Build history of the part. All positions in model axes, mm. Face numbers are marked on the shaded views. A direction names the side the tool comes from. Round coordinates to 2 decimals unless told otherwise and drop trailing zeros. Loops run counter-clockwise (first coordinate to the right, second up) from the corner with the lowest first, then second, coordinate; pieces in that order, holes last.
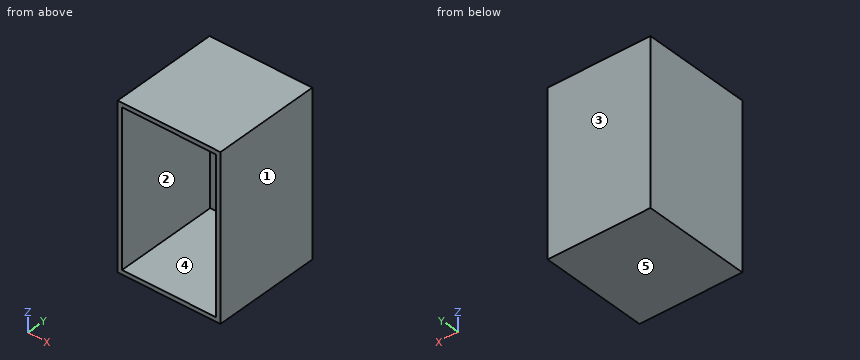
from build123d import *

# Parameters (mm, degrees)
F0_W     = 81.1607763171
F0_H     = 89.4276052713
F1_DEPTH = 381
F2_DEPTH = 482.6
F3_DEPTH = 279.4
F4_T     = -15.24


with BuildPart() as f1:
    # F0 (on Front) → F1 (new body)
    with BuildSketch(Plane.XZ):
        Rectangle(F0_W, F0_H)
    extrude(amount=F1_DEPTH)

    # F2 (add): a face of the model
    f2_faces = [f1.faces().sort_by_distance(p)[0] for p in [
        (0, -190.5, 44.7138026357),
    ]]
    extrude(f2_faces, amount=F2_DEPTH)

    # F3 (add): a face of the model
    f3_faces = [f1.faces().sort_by_distance(p)[0] for p in [
        (40.5803881586, -190.5, 241.3),
    ]]
    extrude(f3_faces, amount=F3_DEPTH)

    # F4
    f4_openings = [f1.faces().sort_by_distance(p)[0] for p in [
        (139.7, -381, 241.3),
    ]]
    offset(amount=F4_T, openings=f4_openings)


solid = f1.part
(1) Slice it at B-B on y = -47. List the corners of the cut face in (x, z), plus the area to 3 significant figures.
Responses:
outline: (-40.58, -44.71) - (319.98, -44.71) - (319.98, 527.31) - (-40.58, 527.31) - close; hole (-25.34, -29.47) - (304.74, -29.47) - (304.74, 512.07) - (-25.34, 512.07) - close
area: 27,500 mm2
(2) Pull direction Z, two halves, no side cores. Call the marked faces 3, 4 and 5: +Z half, -Z half, draft (parallel to the pull), parting line (faces both ways), or undercut.
Responses:
face 3: draft
face 4: undercut
face 5: -Z half
(3) Slice it at A-A on z = 10.5. List the corners of the cut face in (x, y).
Responses:
outline: (-40.58, -381) - (-25.34, -381) - (-25.34, -15.24) - (304.74, -15.24) - (304.74, -381) - (319.98, -381) - (319.98, 0) - (-40.58, 0) - close
(4) Slice it at C-C on x = 64. List the corners of the cut face in (y, z).
Responses:
outline: (-381, -44.71) - (0, -44.71) - (0, 527.31) - (-381, 527.31) - (-381, 512.07) - (-15.24, 512.07) - (-15.24, -29.47) - (-381, -29.47) - close
(5) Which spindle directions (+Z, -Z, +X, -X, +Y, -Y) get a long thin tool onto all of the face, cutting with end or side? Do the marked faces 1 and 2. Say none if no direction does.
Responses:
face 1: +Z, -Z, +X, +Y, -Y
face 2: -Y
(6) Pin check, flat tip, straight feed: P1, Ø1, axis at x = 207, z = 157.5, coming from the -Y side. Stop position of the tip, or through.
Responses:
P1: stops at y = -15.24
(7) Probe line 1 (X direction, y = -279.5, z = 270.5); line 2 (Z direction, x = 185, y = -317); line 3 (Y direction, x = 97, z = 17.5). List the from-to ranges inside material, lowest first.
Responses:
line 1: x = -40.58 to -25.34, 304.74 to 319.98
line 2: z = -44.71 to -29.47, 512.07 to 527.31
line 3: y = -15.24 to 0
